Geometry check sheet. Reference: the model listing, model coordinates, mm. Round coordinates to 2 decimals unless told otherwise and drop trailing zeros. Loops run counter-clockwise (first coordinate to the right, second up) from the corner with the lowest first, then second, coordinate; pieces in that order, holes last.
Autodesk Inventor part; units mm, degrees
ref_plane "Work Plane1" through (0, 0, 0) normal (0.4226, 0.9063, 0) x (0, 0, -1)
ref_plane "Work Plane2" through (10.5655, 22.6577, 0) normal (0.4226, 0.9063, 0) x (0, 0, -1)
ref_plane "YZ Plane" through (0, 0, 0) normal (1, 0, 0) x (0, 1, 0)
sketch "Sketch1" plane through (0, 0, 0) normal (0, 0, 1) x (1, 0, 0)
  circle A0 centre (0, 0) radius 23
  circle A1 centre (0, 0) radius 25
  dimension "d0" = 50
  dimension "d2" = 46
extrude "Extrusion1" add sketch "Sketch1" against normal blind 6
sketch "Sketch2" plane through (0, 0, 0) normal (0, 1, 0) x (-1, 0, 0)
  line L0 (-25, -6) -> (25, -6)
  circle A0 centre (0, -3) radius 1.5
  point P0 (0, 0)
  dimension "d5" = 3
  dimension "d6" = 3
extrude "Extrusion2" cut sketch "Sketch2" along normal through all both and the other way through all
sketch "Sketch3" plane through (0, 0, 0) normal (1, 0, 0) x (0, 1, 0)
  circle A0 centre (0, -3) radius 1.5
  line L0 (-25, 0) -> (25, 0)
  point P0 (0, 0)
  dimension "d9" = 3
  dimension "d10" = 3
extrude "Extrusion3" cut sketch "Sketch3" along normal through all both and the other way through all
ref_plane "Work Plane1" through (0, 0, 0) normal (0.4226, 0.9063, 0) x (0, 0, -1)
ref_plane "Work Plane2" through (10.5655, 22.6577, 0) normal (0.4226, 0.9063, 0) x (0, 0, -1)
sketch "Sketch5" plane through (10.5655, 22.6577, 0) normal (0.4226, 0.9063, 0) x (0, 0, -1)
  circle A0 centre (3, 0) radius 1.5
  line L0 (0, 25) -> (6, 25)
  point P0 (0, 0)
  point P1 (3, 25)
  dimension "d17" = 3
extrude "Extrusion4" cut sketch "Sketch5" against normal blind 10
properties part number "Ball Ring"
1) Scan lines: line 1 along Z through (x, y) = (0, -24.2); line 2 along Y through (x, z) = (-4.5, -2.25); line 3 along Y through (x, z) = (6.5, -5.5). Record each from-to range of solid material in increasing order.
Report:
line 1: z = -6 to -4.5, -1.5 to 0
line 2: y = -24.59 to -22.56, 22.56 to 24.59
line 3: y = -24.14 to -22.06, 22.06 to 24.14
2) Sectioned sample at A-A, the plane x = 0. Record the cut outline in (y, z), then the cut area to 3 significant figures.
Report:
outline: (-25, -6) - (-23, -6) - (-23, -4.5) - (-25, -4.5) - close; (-25, -1.5) - (-23, -1.5) - (-23, 0) - (-25, 0) - close; (23, -6) - (25, -6) - (25, -4.5) - (23, -4.5) - close; (23, -1.5) - (25, -1.5) - (25, 0) - (23, 0) - close
area: 12.0 mm2
3) Mould release check, pull along X, two halves, no side actions. Record for faces 1 (the face through (22.1, -7.3, -6)), 2 (the face through (0.195, -23.961, -1.513)), 3 (the face through (23.846, 7.509, -2.958)): +X half, -X half, draft (parallel to the pull), parting line (faces both ways), or undercut.
Report:
face 1: draft
face 2: undercut
face 3: parting line
4) Sectioned sample at D-D, the plane x = -8. Record the cut outline in (y, z), then the cut area to 3 significant figures.
Report:
outline: (-23.69, -6) - (-21.56, -6) - (-21.56, 0) - (-23.69, 0) - close; (21.56, -6) - (23.69, -6) - (23.69, 0) - (21.56, 0) - close
area: 25.5 mm2
5) Gauge pin test, flat ends, axial feed: pin 1 (1 mm diameter, centred on x = -6, z = -3, fed in from -Y); pin 2 (2 mm diameter, centred on y = 5.5, z = -4.5, fed in from +X); pin 3 (3 mm diameter, centred on x = 10.5, z = -1, fed in from -Y). Record the tip position at first contact, or that the pin passes through.
Report:
pin 1: stops at y = -24.39
pin 2: stops at x = 24.59
pin 3: stops at y = -23.32
6) Sectioned sample at C-C, the plane z = -3. Record the cut outline in (x, y).
Report:
outline: (-24.95, -1.5) arc R25 ccw to (-1.5, -24.95) - (-1.5, -22.95) arc R23 cw to (-22.95, -1.5) - close; (-24.95, 1.5) - (-22.95, 1.5) arc R23 cw to (-1.5, 22.95) - (-1.5, 24.95) arc R25 ccw to start; (1.5, -24.95) arc R25 ccw to (24.95, -1.5) - (22.95, -1.5) arc R23 cw to (1.5, -22.95) - close; (1.5, 22.95) arc R23 cw to (8.34, 21.43) - (9.19, 23.25) arc R25 ccw to (1.5, 24.95) - close; (11.06, 20.17) arc R23 cw to (22.95, 1.5) - (24.95, 1.5) arc R25 ccw to (11.91, 21.98) - close
